Geometry: final body of the model. Coordinates: model frame, mm. A direction names the side the tool comes from. Round coordinates to 2 decimals unless told otherwise and drop trailing zeros. Loops run counter-clockwise (first coordinate to the right, second up) from the corner with the lowest first, then second, coordinate; pieces in that order, holes last. Notation, with made-up numbers: (30.5, 67) - (86.5, 67) arc R22 ccw to (86.5, 86) - close; hole circle Ø7 at (86.5, -5.5). An arc over 180 degrees is marked (long way). Use CSV: the item, a comma, the result in double quotes.
from build123d import *

# Parameters (mm, degrees)
BOSS_EXTRUDE1_DEPTH = 5
BOSS_EXTRUDE2_DEPTH = 40
SKETCH3_R           = 17.5
CUT_EXTRUDE1_DEPTH  = 40
SKETCH4_R           = 26
SKETCH4_R_2         = 23.5
BOSS_EXTRUDE3_DEPTH = 7
SKETCH5_R           = 36
SKETCH5_R_2         = 26
BOSS_EXTRUDE4_DEPTH = 19
BOSS_EXTRUDE5_DEPTH = 17
CUT_EXTRUDE2_DEPTH  = 14
SKETCH8_R           = 1.5
SKETCH8_R_2         = 11
CUT_EXTRUDE3_DEPTH  = 14
SKETCH9_R           = 2.5
CUT_EXTRUDE4_DEPTH  = 45
SKETCH10_R          = 2.5
BOSS_EXTRUDE6_DEPTH = 8


with BuildPart() as part:
    # Sketch1 → Boss-Extrude1 (new body)
    with BuildSketch(Plane(origin=(0, 0, 0), x_dir=(1, 0, 0), z_dir=(0, 1, 0))):
        with BuildLine():
            Line((50, 0), (50, -167.5))
            Line((50, -167.5), (-50, -167.5))
            Line((-50, -167.5), (-50, 0))
            ThreePointArc((-50, 0), (0, 50), (50, 0))
        make_face()
    extrude(amount=BOSS_EXTRUDE1_DEPTH)

    # Sketch2 → Boss-Extrude2 (add)
    with BuildSketch(Plane(origin=(0, 5, 0), x_dir=(1, 0, 0), z_dir=(0, 1, 0))):
        with BuildLine():
            ThreePointArc((50, 0), (0, 50), (-50, 0))
            Line((-50, 0), (-50, -167.5))
            Line((-50, -167.5), (50, -167.5))
            Line((50, -167.5), (50, 0))
        make_face()
        with BuildLine():
            Line((-45, -162.5), (-45, 0))
            ThreePointArc((-45, 0), (0, 45), (45, 0))
            Line((45, 0), (45, -162.5))
            Line((45, -162.5), (-45, -162.5))
        make_face(mode=Mode.SUBTRACT)
    extrude(amount=BOSS_EXTRUDE2_DEPTH)

    # Sketch3 → Cut-Extrude1 (cut)
    with BuildSketch(Plane(origin=(0, 5, 0), x_dir=(1, 0, 0), z_dir=(0, 1, 0))):
        with Locations(Location((0, 0, 0), (0, 0, 270))):
            Circle(SKETCH3_R)
    extrude(amount=-CUT_EXTRUDE1_DEPTH, mode=Mode.SUBTRACT)

    # Sketch4 → Boss-Extrude3 (add)
    with BuildSketch(Plane(origin=(0, 5, 0), x_dir=(1, 0, 0), z_dir=(0, 1, 0))):
        with Locations(Location((0, 0, 0), (0, 0, 90))):
            Circle(SKETCH4_R)
        with Locations(Location((0, 0, 0), (0, 0, 270))):
            Circle(SKETCH4_R_2, mode=Mode.SUBTRACT)
    extrude(amount=BOSS_EXTRUDE3_DEPTH)

    # Sketch5 → Boss-Extrude4 (add)
    with BuildSketch(Plane(origin=(0, 5, 0), x_dir=(1, 0, 0), z_dir=(0, 1, 0))):
        with Locations(Location((0, 0, 0), (0, 0, 90))):
            Circle(SKETCH5_R)
        with Locations(Location((0, 0, 0), (0, 0, 270))):
            Circle(SKETCH5_R_2, mode=Mode.SUBTRACT)
    extrude(amount=BOSS_EXTRUDE4_DEPTH)

    # Sketch6 → Boss-Extrude5 (add)
    with BuildSketch(Plane(origin=(0, 5, 0), x_dir=(1, 0, 0), z_dir=(0, 1, 0))):
        Polygon((24.5, -133), (24.5, -157.5), (-24.5, -157.5), (-24.5, -108.5), (24.5, -108.5), align=None)
    extrude(amount=BOSS_EXTRUDE5_DEPTH)

    # Sketch7 → Cut-Extrude2 (cut)
    with BuildSketch(Plane.XZ):
        Polygon((21.5, 133), (21.5, 154.5), (-21.5, 154.5), (-21.5, 111.5), (21.5, 111.5), align=None)
    extrude(amount=-CUT_EXTRUDE2_DEPTH, mode=Mode.SUBTRACT)

    # Sketch8 → Cut-Extrude3 (cut)
    with BuildSketch(Plane.XZ.offset(-14)):
        with Locations(Location((-15.5, 148.5, 0), (0, 0, 270))):
            Circle(SKETCH8_R)
        with Locations(Location((15.5, 148.5, 0), (0, 0, 270))):
            Circle(SKETCH8_R)
        with Locations(Location((-15.5, 115.5, 0), (0, 0, 270))):
            Circle(SKETCH8_R)
        with Locations(Location((15.5, 115.5, 0), (0, 0, 270))):
            Circle(SKETCH8_R)
        with Locations(Location((0, 133, 0), (0, 0, 270))):
            Circle(SKETCH8_R_2)
    extrude(amount=-CUT_EXTRUDE3_DEPTH, mode=Mode.SUBTRACT)

    # Sketch9 → Cut-Extrude4 (cut)
    with BuildSketch(Plane(origin=(0, 45, 0), x_dir=(1, 0, 0), z_dir=(0, 1, 0))):
        with BuildLine():
            ThreePointArc((-20, -69), (-22.5, -66.5), (-20, -64))
            Line((-20, -64), (-29, -64))
            ThreePointArc((-29, -64), (-31.5, -66.5), (-29, -69))
            Line((-29, -69), (-20, -69))
        make_face()
        with Locations((-20, -66.5)):
            Circle(SKETCH9_R)
        with BuildLine():
            Line((29, -64), (20, -64))
            ThreePointArc((20, -64), (21.767766953, -64.732233047), (22.5, -66.5))
            ThreePointArc((22.5, -66.5), (21.767766953, -68.267766953), (20, -69))
            Line((20, -69), (29, -69))
            ThreePointArc((29, -69), (31.5, -66.5), (29, -64))
        make_face()
        with Locations((20, -66.5)):
            Circle(SKETCH9_R)
    extrude(amount=-CUT_EXTRUDE4_DEPTH, mode=Mode.SUBTRACT)

    # Sketch10 → Boss-Extrude6 (add)
    # profile 1 of 8: a face of its own
    with BuildSketch(Plane(origin=(0, 45, 0), x_dir=(1, 0, 0), z_dir=(0, 1, 0))):
        with BuildLine():
            Line((-54, -70), (-50, -70))
            Line((-50, -70), (-50, -63))
            Line((-50, -63), (-54, -63))
            ThreePointArc((-54, -63), (-57.5, -66.5), (-54, -70))
        make_face()
        with Locations(Location((-54, -66.5, 0), (0, 0, 270))):
            Circle(SKETCH10_R, mode=Mode.SUBTRACT)
    # profile 2 of 8: a face of its own
    with BuildSketch(Plane(origin=(0, 45, 0), x_dir=(1, 0, 0), z_dir=(0, 1, 0))):
        with BuildLine():
            Line((-54, -7), (-50, -7))
            Line((-50, -7), (-50, 0))
            Line((-50, 0), (-54, 0))
            ThreePointArc((-54, 0), (-57.5, -3.5), (-54, -7))
        make_face()
        with Locations(Location((-54, -3.5, 0), (0, 0, 270))):
            Circle(SKETCH10_R, mode=Mode.SUBTRACT)
    # profile 3 of 8: a face of its own
    with BuildSketch(Plane(origin=(0, 45, 0), x_dir=(1, 0, 0), z_dir=(0, 1, 0))):
        with BuildLine():
            Line((-54, -136), (-50, -136))
            Line((-50, -136), (-50, -130))
            Line((-50, -130), (-54, -130))
            ThreePointArc((-54, -130), (-57, -133), (-54, -136))
        make_face()
        with Locations(Location((-54, -133, 0), (0, 0, 270))):
            Circle(SKETCH10_R, mode=Mode.SUBTRACT)
    # profile 4 of 8: a face of its own
    with BuildSketch(Plane(origin=(0, 45, 0), x_dir=(1, 0, 0), z_dir=(0, 1, 0))):
        with BuildLine():
            Line((28, -171.5), (28, -167.5))
            Line((28, -167.5), (21, -167.5))
            Line((21, -167.5), (21, -171.5))
            ThreePointArc((21, -171.5), (24.5, -175), (28, -171.5))
        make_face()
        with Locations(Location((24.5, -171.5, 0), (0, 0, 270))):
            Circle(SKETCH10_R, mode=Mode.SUBTRACT)
    # profile 5 of 8: a face of its own
    with BuildSketch(Plane(origin=(0, 45, 0), x_dir=(1, 0, 0), z_dir=(0, 1, 0))):
        with BuildLine():
            Line((-21, -171.5), (-21, -167.5))
            Line((-21, -167.5), (-28, -167.5))
            Line((-28, -167.5), (-28, -171.5))
            ThreePointArc((-28, -171.5), (-24.5, -175), (-21, -171.5))
        make_face()
        with Locations(Location((-24.5, -171.5, 0), (0, 0, 270))):
            Circle(SKETCH10_R, mode=Mode.SUBTRACT)
    # profile 6 of 8: a face of its own
    with BuildSketch(Plane(origin=(0, 45, 0), x_dir=(1, 0, 0), z_dir=(0, 1, 0))):
        with BuildLine():
            Line((54, -129.5), (50, -129.5))
            Line((50, -129.5), (50, -136.5))
            Line((50, -136.5), (54, -136.5))
            ThreePointArc((54, -136.5), (57.5, -133), (54, -129.5))
        make_face()
        with Locations(Location((54, -133, 0), (0, 0, 270))):
            Circle(SKETCH10_R, mode=Mode.SUBTRACT)
    # profile 7 of 8: a face of its own
    with BuildSketch(Plane(origin=(0, 45, 0), x_dir=(1, 0, 0), z_dir=(0, 1, 0))):
        with BuildLine():
            Line((54, -63), (50, -63))
            Line((50, -63), (50, -70))
            Line((50, -70), (54, -70))
            ThreePointArc((54, -70), (57.5, -66.5), (54, -63))
        make_face()
        with Locations(Location((54, -66.5, 0), (0, 0, 270))):
            Circle(SKETCH10_R, mode=Mode.SUBTRACT)
    # profile 8 of 8: a face of its own
    with BuildSketch(Plane(origin=(0, 45, 0), x_dir=(1, 0, 0), z_dir=(0, 1, 0))):
        with BuildLine():
            Line((54, 0), (50, 0))
            Line((50, 0), (50, -7))
            Line((50, -7), (54, -7))
            ThreePointArc((54, -7), (57.5, -3.5), (54, 0))
        make_face()
        with Locations(Location((54, -3.5, 0), (0, 0, 270))):
            Circle(SKETCH10_R, mode=Mode.SUBTRACT)
    extrude(amount=-BOSS_EXTRUDE6_DEPTH)


solid = part.part
Item 1: Mould query, pull axis Z, two halves, no side actions, for faces 1 (the flat face through (45, 25, 80)), 2 (the flat face through (52, 41, 0)), 3 (the flat face through (52, 41, 136.5)). Classes: released by +Z, released by -Z, zero draft, split by the parting line, or undercut.
Final values:
face 1,"undercut"
face 2,"released by -Z"
face 3,"released by +Z"
Item 2: Pin query (flat end, axial travel): P1, Ø8, axis at x = 44.5, y = 39.5, coming from the -Z side; P2, Ø1, axis at x = -10.5, y = 23.5, coming from the +Z side; P3, Ø2, axis at x = 51.5, y = 39.5, coming from the +Z side. Return the tip coordinate at first contact, or that it passes through.
Final values:
P1,"stops at z = -29.32"
P2,"stops at z = 167.5"
P3,"stops at z = 136.5"
Item 3: Section C-C on z = 95. Return the cut outline in (x, y), plus the area to 3 significant figures.
Final values:
outline,"(-50, 0) - (50, 0) - (50, 45) - (45, 45) - (45, 5) - (-45, 5) - (-45, 45) - (-50, 45) - close"
area,"900 mm²"
Item 4: Section B-B on y = 28. Return the cut outline in (x, z), plus the area to 3 significant figures.
Final values:
outline,"(-50, 0) arc R50 ccw to (50, 0) - (50, 167.5) - (-50, 167.5) - close; hole (-45, 0) arc R45 ccw to (45, 0) - (45, 162.5) - (-45, 162.5) - close"
area,"2,870 mm²"
Item 5: Material intervals for line 1 (X direction, y = 21, z = 153); line 2 (X direction, y = 7.5, z = 135); line 3 (X direction, y = 18.75, z = 0), sorted ascending.
Final values:
line 1,"x = -50 to -45, -24.5 to 24.5, 45 to 50"
line 2,"x = -50 to -45, -24.5 to -21.5, 21.5 to 24.5, 45 to 50"
line 3,"x = -50 to -45, -36 to -26, 26 to 36, 45 to 50"
Item 6: Section A-A on z = 66.5. Return the cut outline in (x, y), plus the area to 3 significant figures.
Final values:
outline,"(-57.5, 37) - (-56.5, 37) - (-56.5, 45) - (-57.5, 45) - close; (-51.5, 37) - (-50, 37) - (-50, 0) - (-31.5, 0) - (-31.5, 5) - (-45, 5) - (-45, 45) - (-51.5, 45) - close; (-17.5, 0) - (17.5, 0) - (17.5, 5) - (-17.5, 5) - close; (31.5, 0) - (50, 0) - (50, 37) - (51.5, 37) - (51.5, 45) - (45, 45) - (45, 5) - (31.5, 5) - close; (56.5, 37) - (57.5, 37) - (57.5, 45) - (56.5, 45) - close"
area,"800 mm²"
Item 7: Reachability of faces 4 (the flat face through (-21.5, 7, 133)), 5 (the flat face through (-52, 41, 130)), 6 (the flat face through (24.5, 13, 133)) from +Z, -Z, +X, -X, +Y, -Y: full face, straight path, thin tool, end or side. Return the list, or none.
Final values:
face 4,"-Y"
face 5,"-X, +Y, -Y"
face 6,"+Y"
Item 8: Section D-D on x = 0. Give the number of separate pieces and of enclosed holes in the cut face, plus the area to 3 significant figures.
Final values:
separate pieces,"3"
enclosed holes,"0"
area,"1,780 mm²"
